Input: part model. Units: mm. Frame: model coordinates. A direction names the side the tool comes from. Coordinates: 2 decimals unless noted, no trailing zeros. Write each loop counter-clockwise with the first axis right and the second up, starting at its lowest first coordinate (ties: lowest second). Pieces come first, ordered by that corner, then holes. Notation, with made-up numbers: (17, 64.25) - (43, 64.25) arc R16 cw to (43, 81.25) - close; hole circle Ø7 at (41, -8.5). An arc over 180 degrees is marked (long way). Use a Markdown table: item, result. Add a question column.
Q1. Pin query (flat end, axial travel): P1, Ø3, axis at y = -12, z = 12, coming from the -X side; P2, Ø2, axis at y = 7, z = 13.5, coming from the +X side; P3, Ø3, axis at x = -65, y = -86.5, coming from the +Z side. Return the tip coordinate at first contact, or that it passes through.
Q2. Material intervals for probe 1 along Y at (x, z) = (47, 7); probe 2 along X at (y, z) = (1.5, 21.75), sorted ascending. Write a range as from..to.
Q3. Mould query, pull axis Y, two halves, no side actions, for faces 1 (the face through (-1, 1, 24)), 2 (the face through (-68, -92.781, 17)), 3 (the face through (-1, -95, 12)), 4 (the face through (-45, 77.5, 12)). Classes: released by +Y, released by -Y, zero draft, split by the parting line, or undercut.
Q4. Section query A-A (x = 29). Return the cut outline in (y, z), then the cut area to 3 significant figures.
Q5. Section query C-C (y = 86.25). Return the cut outline in (x, z), then the cut area to 3 significant figures.
Q6. Set-up query: faces 5 (the face through (-19, -1, 12)), 6 (the face through (68, -92.781, 17)), 7 (the face through (-68, 79.719, 17)), 8 (the face through (44, -77.5, 12)). Return all of +Z, -Z, +X, -X, +Y, -Y with unobstructed straight access to the full face (end or side cutting, diameter ignored); none if empty.
Q7. Section query B-B (z = 12.75). Return the cut outline in (x, y), then the cut area to 3 significant figures.
Q8. Section query D-D (y = 60.5). Return the cut outline in (x, z).
from build123d import *

# Parameters (mm, degrees)
SKETCH1_W           = 35
SKETCH1_H           = 155
SKETCH1_H_2         = 17.5
BOSS_EXTRUDE1_DEPTH = 24
SKETCH2_W           = 51
SKETCH2_H           = 77.5
CUT_EXTRUDE1_DEPTH  = 24
CUT_EXTRUDE2_DEPTH  = 14


with BuildPart() as part:
    # Sketch1 → Boss-Extrude1 (new body)
    with BuildSketch(Plane.XY):
        with Locations((-52.5, 0)):
            Rectangle(SKETCH1_W, SKETCH1_H)
        with Locations((-52.5, 86.25)):
            Rectangle(SKETCH1_W, SKETCH1_H_2)
        Polygon((35, 95), (-35, 95), (-35, 77.5), (-35, -77.5), (-35, -95), (35, -95), (35, -77.5), (35, 77.5), align=None)
        with Locations((52.5, 86.25)):
            Rectangle(SKETCH1_W, SKETCH1_H_2)
        with Locations((52.5, 0)):
            Rectangle(SKETCH1_W, SKETCH1_H)
        with Locations((52.5, -86.25)):
            Rectangle(SKETCH1_W, SKETCH1_H_2)
        with Locations((-52.5, -86.25)):
            Rectangle(SKETCH1_W, SKETCH1_H_2)
    extrude(amount=BOSS_EXTRUDE1_DEPTH)

    # Sketch2 → Cut-Extrude1 (cut)
    with BuildSketch(Plane.XY.offset(24)):
        with Locations((-44.5, 38.75)):
            Rectangle(SKETCH2_W, SKETCH2_H)
        with Locations((-44.5, -38.75)):
            Rectangle(SKETCH2_W, SKETCH2_H)
        Polygon((35, 77.5), (19, 77.5), (19, 0), (70, 0), (70, 77.5), align=None)
        Polygon((70, 0), (19, 0), (19, -77.5), (35, -77.5), (70, -77.5), align=None)
    extrude(amount=-CUT_EXTRUDE1_DEPTH, mode=Mode.SUBTRACT)

    # Sketch3 → Cut-Extrude2 (cut)
    with BuildSketch(Plane.XY.offset(24)):
        with BuildLine():
            Line((70, -92.781156562), (66, -92.781156562))
            ThreePointArc((66, -92.781156562), (59.468843438, -86.25), (66, -79.718843438))
            Line((66, -79.718843438), (70, -79.718843438))
            ThreePointArc((70, -79.718843438), (76.531156562, -86.25), (70, -92.781156562))
        make_face()
        with BuildLine():
            Line((70, 92.781156562), (66, 92.781156562))
            ThreePointArc((66, 92.781156562), (59.468843438, 86.25), (66, 79.718843438))
            Line((66, 79.718843438), (70, 79.718843438))
            ThreePointArc((70, 79.718843438), (76.531156562, 86.25), (70, 92.781156562))
        make_face()
        with BuildLine():
            Line((-70, 92.781156562), (-66, 92.781156562))
            ThreePointArc((-66, 92.781156562), (-59.468843438, 86.25), (-66, 79.718843438))
            Line((-66, 79.718843438), (-70, 79.718843438))
            ThreePointArc((-70, 79.718843438), (-76.531156562, 86.25), (-70, 92.781156562))
        make_face()
        with BuildLine():
            Line((-70, -92.781156562), (-66, -92.781156562))
            ThreePointArc((-66, -92.781156562), (-59.468843438, -86.25), (-66, -79.718843438))
            Line((-66, -79.718843438), (-70, -79.718843438))
            ThreePointArc((-70, -79.718843438), (-76.531156562, -86.25), (-70, -92.781156562))
        make_face()
    extrude(amount=-CUT_EXTRUDE2_DEPTH, mode=Mode.SUBTRACT)


solid = part.part
Values follow:
| question | item | result |
|---|---|---|
| 1 | P1 | x = -19 |
| 1 | P2 | x = 19 |
| 1 | P3 | z = 10 |
| 2 | probe 1 | -95..-77.5, 77.5..95 |
| 2 | probe 2 | -19..19 |
| 3 | face 1 | zero draft |
| 3 | face 2 | undercut |
| 3 | face 3 | released by -Y |
| 3 | face 4 | undercut |
| 4 | outline | (-95, 0) - (-77.5, 0) - (-77.5, 24) - (-95, 24) - close; (77.5, 0) - (95, 0) - (95, 24) - (77.5, 24) - close |
| 4 | area | 840 mm2 |
| 5 | outline | (-70, 0) - (70, 0) - (70, 10) - (59.47, 10) - (59.47, 24) - (-59.47, 24) - (-59.47, 10) - (-70, 10) - close |
| 5 | area | 3,070 mm2 |
| 6 | face 5 | +Z, -Z, -X |
| 6 | face 6 | +Z, +X |
| 6 | face 7 | +Z, -X |
| 6 | face 8 | +Z, -Z, +X |
| 7 | outline | (-70, -95) - (70, -95) - (70, -92.78) - (66, -92.78) arc R6.53 cw to (66, -79.72) - (70, -79.72) - (70, -77.5) - (19, -77.5) - (19, 77.5) - (70, 77.5) - (70, 79.72) - (66, 79.72) arc R6.53 cw to (66, 92.78) - (70, 92.78) - (70, 95) - (-70, 95) - (-70, 92.78) - (-66, 92.78) arc R6.53 cw to (-66, 79.72) - (-70, 79.72) - (-70, 77.5) - (-19, 77.5) - (-19, -77.5) - (-70, -77.5) - (-70, -79.72) - (-66, -79.72) arc R6.53 cw to (-66, -92.78) - (-70, -92.78) - close |
| 7 | area | 10,300 mm2 |
| 8 | outline | (-19, 0) - (19, 0) - (19, 24) - (-19, 24) - close |
